Job drawing, mm, ordinate dimensions from the low corner. One solid piece. A direction names the side the tool comes from. Give positions to 0.01 mm unless a question says otherwise; leave off trailing zeros. Order: outer loops, then holes, each group sorted by start corner. A loop starts at its lowest first (then second) coordinate and runs counter-clockwise, first axis right, second up. Notation, with made-up numbers: M -20.75,76.25 L 32.25,76.25 A19 cw 32.25,89.25 Z; hole C 39.5,49.25 d11. An arc over 180 degrees is marked long. One line per question, with ' | ' between items.
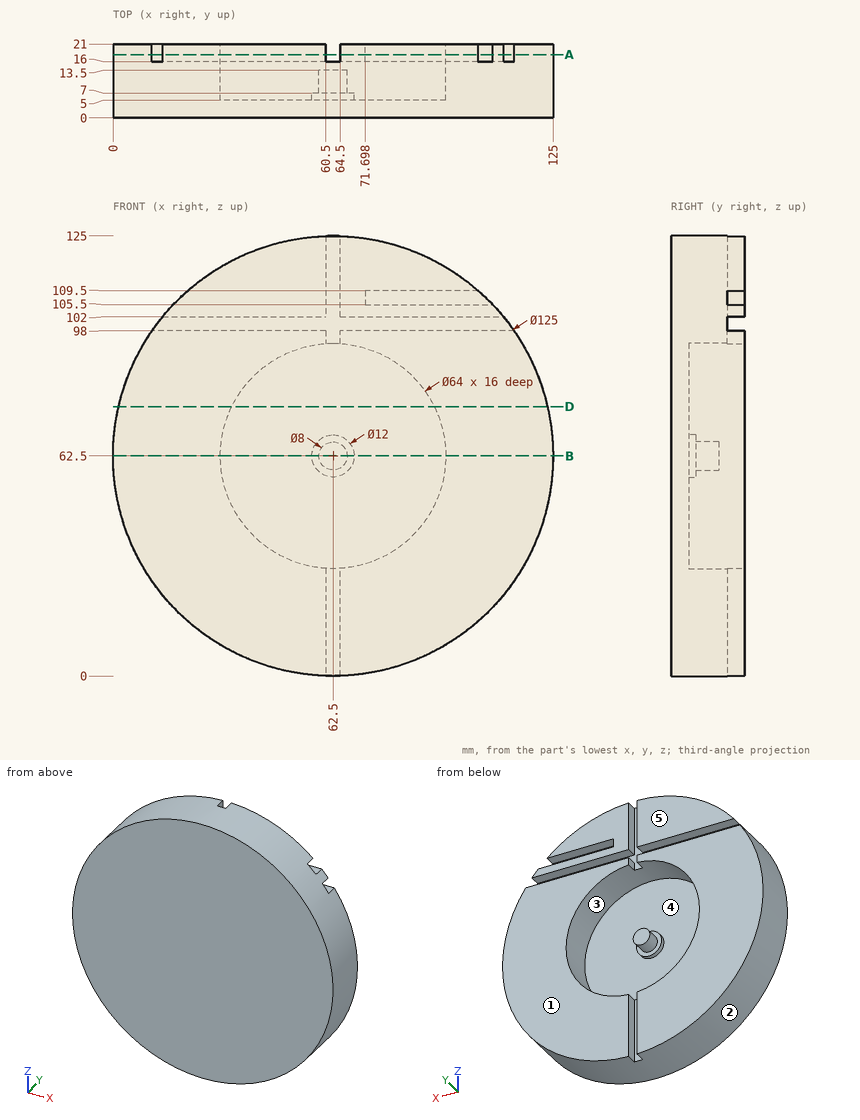
1. Drop flat-ended pins along their axis: pin 1 (1.2 mm diameter, centred on y = 19, z = 107.5, fed in from +X); pin 2 (1.5 mm diameter, centred on y = 17.5, z = 22.5, fed in from -X); pin 3 (5.5 mm diameter, centred on x = 94.5, y = 17.5, fed in from +Z). Give the stop position or say it passes through.
Worked out:
pin 1: stops at x = 71.7 | pin 2: stops at x = 13.86 | pin 3: stops at z = 117.73
2. Mould opens along Z. For the marked faces 1, 2 and 3 say: released by +Z, released by -Z, zero draft, split by the parting line, or undercut.
Worked out:
face 1: zero draft | face 2: split by the parting line | face 3: undercut
3. Probe L1, parallel to X at y = 12.75, z = 62.5; L2, parallel to X at y = 16.25, z = 62.5; L3, parallel to Z at x = 37.5, y = 17 (1 decimal). List the from-to ranges inside material, lowest first. Write a range as from..to.
Worked out:
L1: x = 0..30.5, 58.5..66.5, 94.5..125 | L2: x = 0..30.5, 94.5..125 | L3: z = 5.2..42.5, 82.5..98, 102..119.8
4. Slice it at D-D on z = 76.5. Give the cut face in (x, y) (1 decimal).
Worked out:
outline: M 1.6,0 L 123.4,0 L 123.4,21 L 91.3,21 L 91.3,5 L 33.7,5 L 33.7,21 L 1.6,21 Z
5. Slice it at B-B on z = 62.5. Give the cut face in (x, y), then the cut area to 3 significant figures.
Worked out:
outline: M 0,0 L 125,0 L 125,21 L 94.5,21 L 94.5,5 L 68.5,5 L 68.5,7 L 66.5,7 L 66.5,13.5 L 58.5,13.5 L 58.5,7 L 56.5,7 L 56.5,5 L 30.5,5 L 30.5,21 L 0,21 Z | area: 1,680 mm2
6. Slice it at A-A on y = 18. Give the cut face in (x, z) (1 decimal), then the cut area to 3 significant figures.
Worked out:
outline: M 11.1,98 A62.5 ccw 60.5,0 L 60.5,30.6 A32 cw 60.5,94.4 L 60.5,98 Z; M 14.1,102 L 60.5,102 L 60.5,125 A62.5 ccw Z; M 64.5,0 A62.5 ccw 113.9,98 L 64.5,98 L 64.5,94.4 A32 cw 64.5,30.6 Z; M 64.5,102 L 110.9,102 A62.5 ccw 107.9,105.5 L 71.7,105.5 L 71.7,109.5 L 103.7,109.5 A62.5 ccw 64.5,125 Z | area: 8,290 mm2
7. Tool access for the marked faces 4 and 5: list every direction of +Z, -Z, +X, -X, +Y, -Y with a clear straight run to the whole face (end or side of a thin tool).
Worked out:
face 4: +Y | face 5: +Z, -Z, +X, -X, +Y
